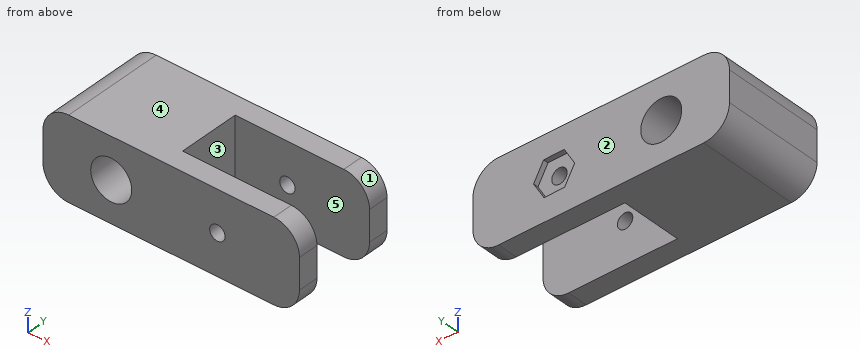
from build123d import *

# Parameters (mm, degrees)
F0_W      = 50
F0_H      = 16
F2_DEPTH  = 20
F3_D      = 8
F3_DEPTH  = 20
F5_D      = 3
F5_DEPTH  = 20
F7_DEPTH  = 26.2
F8_R      = 5
F10_DEPTH = 1


with BuildPart() as f2:
    # F0 (on Front) → F2 (new body)
    with BuildSketch(Plane.XZ):
        Rectangle(F0_W, F0_H)
    extrude(amount=F2_DEPTH)

    # F3
    with Locations(Plane(origin=(0, 0, 0), x_dir=(1, 0, 0), z_dir=(0, 1, 0))):
        with Locations((-11.699282, 0)):
            Hole(F3_D / 2, depth=F3_DEPTH)

    # F5
    with Locations(Plane.XZ.offset(20)):
        with Locations((9, 0)):
            Hole(F5_D / 2, depth=F5_DEPTH)

    # F6 (on face) → F7 (cut)
    with BuildSketch(Plane.YZ.offset(25)):
        Polygon((-16, 8), (-16, 0), (-16, -8), (-4, -8), (-4, 0), (-4, 8), align=None)
    extrude(amount=-F7_DEPTH, mode=Mode.SUBTRACT)

    # F8
    f8_edges = [f2.edges().sort_by_distance(p)[0] for p in [
        (25, -18, 8),
        (25, -2, 8),
        (25, -2, -8),
        (25, -18, -8),
        (-25, -10, -8),
        (-25, -10, 8),
    ]]
    fillet(f8_edges, radius=F8_R)

    # F9 (on Front) → F10 (cut)
    with BuildSketch(Plane.XZ):
        Polygon((11.143559, -3.499542), (13.194126, -0.052143), (11.233874, 3.447399), (7.223055, 3.499542), (5.172489, 0.052143), (7.132741, -3.447399), align=None)
    extrude(amount=F10_DEPTH, mode=Mode.SUBTRACT)


solid = f2.part
Check sheet for the modelled part. Datum: model origin and axes. Units: mm. Face numbers are marked on the shaded views. A direction names the side the tool comes from. Round coordinates to 2 decimals unless told otherwise and drop trailing zeros. Loops run counter-clockwise (first coordinate to the right, second up) from the corner with the lowest first, then second, coordinate; pieces in that order, holes last. Notation, with made-up numbers: M 32,-37.5 L 69,-37.5 A9 cw 69,-31.5 Z; hole C -0.5,1.25 d10. An arc over 180 degrees is marked long. One line per item, written item: value.
(1) Sectioned sample at A-A, the plane y = -11.25. Record the cut outline in (x, z).
Computed values:
outline: M -25,-3 A5 ccw -20,-8 L -1.2,-8 L -1.2,8 L -20,8 A5 ccw -25,3 Z; hole C -11.7,0 d8
(2) Sectioned sample at D-D, the plane x = 9. Record the cut outline in (y, z), then the cut area to 3 significant figures.
Computed values:
outline: M -20,-8 L -16,-8 L -16,-1.5 L -20,-1.5 Z; M -20,1.5 L -16,1.5 L -16,8 L -20,8 Z; M -4,-8 L 0,-8 L 0,-3.47 L -1,-3.47 L -1,-1.5 L -4,-1.5 Z; M -4,1.5 L -1,1.5 L -1,3.48 L 0,3.48 L 0,8 L -4,8 Z
area: 100 mm^2
(3) Release check for a two-part mould opening along Y. For the marked faces 1, 2 and 3 record: +Y half, -Y half, draft (parallel to the pull), parting line (faces both ways), or undercut.
Computed values:
face 1: draft
face 2: +Y half
face 3: undercut
(4) Depth check by flat-ended pin: pin 1 Ø4 at (x, z) = (9, 0) entering from +Y. Enter the tip coordinate at first touch or a pass-through.
Computed values:
pin 1: stops at y = -1
(5) Thickness scan on line 1 (Z direction, x = 9, y = -18.55); line 2 (Y direction, x = 10.5, z = -1); line 3 (Y direction, x = 22, z = 4.5). Record the ranges inside material, lowest first.
Computed values:
line 1: z = -8 to -1.5, 1.5 to 8
line 2: y = -20 to -16, -4 to -1
line 3: y = -20 to -16, -4 to 0
(6) Access from +Z, -Z, +X, -X, +Y, -Y to the whole of each face (thin tool, end or side, straight path). Record for the marked faces 4 and 5.
Computed values:
face 4: +Z, +X, -X, +Y, -Y
face 5: +Z, -Z, +X
(7) Sectioned sample at C-C, the plane x = 15. Record the cut outline in (y, z), then the cut area to 3 significant figures.
Computed values:
outline: M -20,-8 L -16,-8 L -16,8 L -20,8 Z; M -4,-8 L 0,-8 L 0,8 L -4,8 Z
area: 128 mm^2
(8) Sectioned sample at B-B, the plane z = -1. Record the cut outline in (x, y), then the cut area to 3 significant figures.
Computed values:
outline: M -25,-20 L -15.57,-20 L -15.57,0 L -25,0 Z; M -7.83,-20 L 7.88,-20 L 7.88,-16 L -1.2,-16 L -1.2,-4 L 7.88,-4 L 7.88,-1 L 5.76,-1 L 5.76,0 L -7.83,0 Z; M 10.12,-20 L 25,-20 L 25,-16 L 10.12,-16 Z; M 10.12,-4 L 25,-4 L 25,0 L 12.63,0 L 12.63,-1 L 10.12,-1 Z
area: 508 mm^2
